Work out the finished part from the listing and answer in its coordinate system (mm). Coordinates: 2 decimals unless noted, no trailing zeros. Order: outer loops, then holes, each group sorted by start corner. A loop starts at its lowest first (then second) coordinate and runs counter-clockwise, first axis right, second up. Notation, with made-up numbers: (-30.5, 21.5) -> (8.5, 21.5) arc R36 ccw to (8.5, 60.5) -> close; hole circle Ø10 at (75, 52.5). An arc over 180 degrees is marked (long way). Write item = value, one per line. Start each with the question number.
Q1. Flat-ended cylindrical pins translate along their axes: pin 1 (1 mm diameter, centred on x = -20.5, z = 1.5, fed in from +Y); pin 2 (6.5 mm diameter, centred on x = -91.92, y = 91.92, fed in from +Z). Find the tip coordinate at first contact, or state that the pin passes through.
Q2. The part is cut by section A-A, the plane y = -83.5. Determine the outline of the cut face in (x, z) (3 decimals), plus the area to 3 significant figures.
Q3. The part is cut by section C-C, the plane y = 2. Determine the outline of the cut face in (x, z).
Q4. The part is cut by section B-B, the plane z = 3.85. Count the separate pieces of the cut face and the enclosed holes in it, plus the area to 3 significant figures.
Q5. Straight lines are drawn through the part: L1, parallel to Y at x = 82, z = 2.6; L2, parallel to Y at x = -91.5, z = 3.5; L3, parallel to Y at x = 6, z = 1.75. For each, find the intervals that lie inside material, in ascending order. Write a range as from..to.
```python
from build123d import *

# Parameters (mm, degrees)
SKETCH1_R           = 2
SKETCH1_R_2         = 1.95
SKETCH1_R_3         = 1.5
BOSS_EXTRUDE1_DEPTH = 5


with BuildPart() as part:
    # Sketch1 → Boss-Extrude1 (new body)
    with BuildSketch(Plane.XY):
        with BuildLine():
            Line((-90, 100), (-70, 100))
            Line((-70, 100), (-14.884168151, 68.505238943))
            ThreePointArc((-14.884168151, 68.505238943), (0, 64.552533207), (14.884168151, 68.505238943))
            Line((14.884168151, 68.505238943), (70, 100))
            Line((70, 100), (90, 100))
            ThreePointArc((90, 100), (97.071067812, 97.071067812), (100, 90))
            Line((100, 90), (100, 29))
            Line((100, 29), (93.372317414, 9.7797205))
            ThreePointArc((93.372317414, 9.7797205), (91.733506862, 0), (93.372317414, -9.7797205))
            Line((93.372317414, -9.7797205), (100, -29))
            Line((100, -29), (100, -90))
            ThreePointArc((100, -90), (97.071067812, -97.071067812), (90, -100))
            Line((90, -100), (70, -100))
            Line((70, -100), (14.884168151, -68.505238943))
            ThreePointArc((14.884168151, -68.505238943), (0, -64.552533207), (-14.884168151, -68.505238943))
            Line((-14.884168151, -68.505238943), (-70, -100))
            Line((-70, -100), (-90, -100))
            ThreePointArc((-90, -100), (-97.071067812, -97.071067812), (-100, -90))
            Line((-100, -90), (-100, -29))
            Line((-100, -29), (-93.372317414, -9.7797205))
            ThreePointArc((-93.372317414, -9.7797205), (-91.733506862, 0), (-93.372317414, 9.7797205))
            Line((-93.372317414, 9.7797205), (-100, 29))
            Line((-100, 29), (-100, 90))
            ThreePointArc((-100, 90), (-97.071067812, 97.071067812), (-90, 100))
        make_face()
        with Locations((-91.923881554, 91.923881554)):
            Circle(SKETCH1_R, mode=Mode.SUBTRACT)
        with Locations((91.923881554, 91.923881554)):
            Circle(SKETCH1_R, mode=Mode.SUBTRACT)
        with Locations((91.923881554, -91.923881554)):
            Circle(SKETCH1_R, mode=Mode.SUBTRACT)
        with Locations((-91.923881554, -91.923881554)):
            Circle(SKETCH1_R, mode=Mode.SUBTRACT)
        with Locations((58, 29)):
            Circle(SKETCH1_R_2, mode=Mode.SUBTRACT)
        with Locations((82, 29)):
            Circle(SKETCH1_R_2, mode=Mode.SUBTRACT)
        with Locations((58, 11)):
            Circle(SKETCH1_R_2, mode=Mode.SUBTRACT)
        with Locations((82, 11)):
            Circle(SKETCH1_R_2, mode=Mode.SUBTRACT)
        with Locations((58, -11)):
            Circle(SKETCH1_R_2, mode=Mode.SUBTRACT)
        with Locations((58, -29)):
            Circle(SKETCH1_R_2, mode=Mode.SUBTRACT)
        with Locations((82, -11)):
            Circle(SKETCH1_R_2, mode=Mode.SUBTRACT)
        with Locations((82, -29)):
            Circle(SKETCH1_R_2, mode=Mode.SUBTRACT)
        with Locations((-82, 29)):
            Circle(SKETCH1_R_2, mode=Mode.SUBTRACT)
        with Locations((-58, 29)):
            Circle(SKETCH1_R_2, mode=Mode.SUBTRACT)
        with Locations((-82, 11)):
            Circle(SKETCH1_R_2, mode=Mode.SUBTRACT)
        with Locations((-58, 11)):
            Circle(SKETCH1_R_2, mode=Mode.SUBTRACT)
        with Locations((-82, -11)):
            Circle(SKETCH1_R_2, mode=Mode.SUBTRACT)
        with Locations((-82, -29)):
            Circle(SKETCH1_R_2, mode=Mode.SUBTRACT)
        with Locations((-58, -11)):
            Circle(SKETCH1_R_2, mode=Mode.SUBTRACT)
        with Locations((-58, -29)):
            Circle(SKETCH1_R_2, mode=Mode.SUBTRACT)
        with Locations((-6, 10)):
            Circle(SKETCH1_R_3, mode=Mode.SUBTRACT)
        with Locations((6, 10)):
            Circle(SKETCH1_R_3, mode=Mode.SUBTRACT)
        with Locations((-6, -10)):
            Circle(SKETCH1_R_3, mode=Mode.SUBTRACT)
        with Locations((6, -10)):
            Circle(SKETCH1_R_3, mode=Mode.SUBTRACT)
    extrude(amount=BOSS_EXTRUDE1_DEPTH)


solid = part.part
```
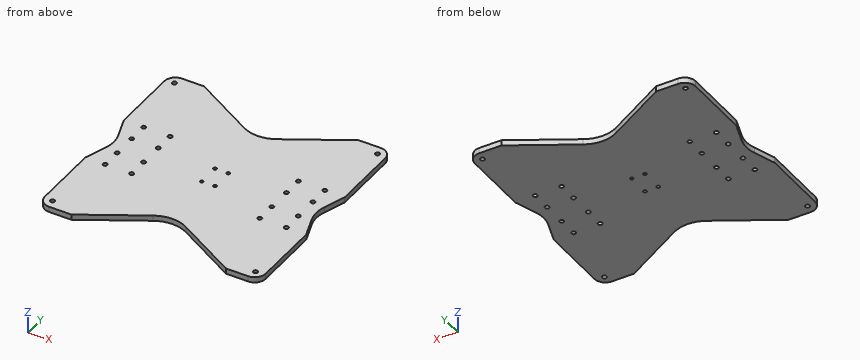
Model answer:
q1.pin_1 = 72
q1.pin_2 = 5
q2.outline = (-100, 0) -> (-41.125, 0) -> (-41.125, 5) -> (-100, 5) -> close; (41.125, 0) -> (100, 0) -> (100, 5) -> (41.125, 5) -> close
q2.area = 589 mm2
q3.outline = (-91.8, 0) -> (91.8, 0) -> (91.8, 5) -> (-91.8, 5) -> close
q4.separate_pieces = 1
q4.enclosed_holes = 24
q4.area = 33,600 mm2
q5.L1 = -100..-30.95, -27.05..-12.95, -9.05..9.05, 12.95..27.05, 30.95..100
q5.L2 = -99.89..-93.88, -89.97..89.97, 93.88..99.89
q5.L3 = -65.16..-11.5, -8.5..8.5, 11.5..65.16
